Study the drawing (mm; zero at the part's minimum x, y, z) and answer. A direction names the side the tool comes from. Coordinates: 2 decimals unless noted, no trailing zeros. Order: outer loops, then holes, each group sorted by start corner. A loop starts at its lowest first (then second) coordinate and runs counter-clockwise, first axis right, second up. Notation, with made-up numbers: (54.25, 64) -> (69.25, 64) arc R16 cw to (69.25, 74) -> close; hole circle Ø10 at (34, -16). An arc over 180 degrees is marked (long way). Answer as CSV lines item,"result". Start each with the question number.
Item 1: Section A-A (z = 33) is taken. Write down the section's boundary in (x, y).
Item 2: Section B-B (y = 6) is taken. Write down the section's boundary in (x, z).
Item 3: Which of the six approach directions +Z, -Z, +X, -X, +Y, -Y give full straight-line access (tool end or side, diameter ignored) to the marked faces 1 and 2?
Item 4: Straight lines are drawn through the part: L1, parallel to X at y = 7.75, z = 28; L2, parallel to Z at x = 66.5, y = 6.75; L3, parallel to X at y = 6, z = 43.5. For each, find the intervals that lie inside material, in ascending order.
Item 5: Section C-C (x = 39) is taken. Write down the section's boundary in (y, z).
Item 6: Each of these flat-tipped pins is pushed along its axis until it touches: pin 1 Ø1.5 at (y, z) = (8, 35.5) entering from -X; pin 2 Ø3 at (y, z) = (10, 8.5) entering from -X. Where does it stop, or does it pass through?
Item 7: Section D-D (z = 44) is taken. Write down the section's boundary in (x, y), then the cut area to 3 significant figures.
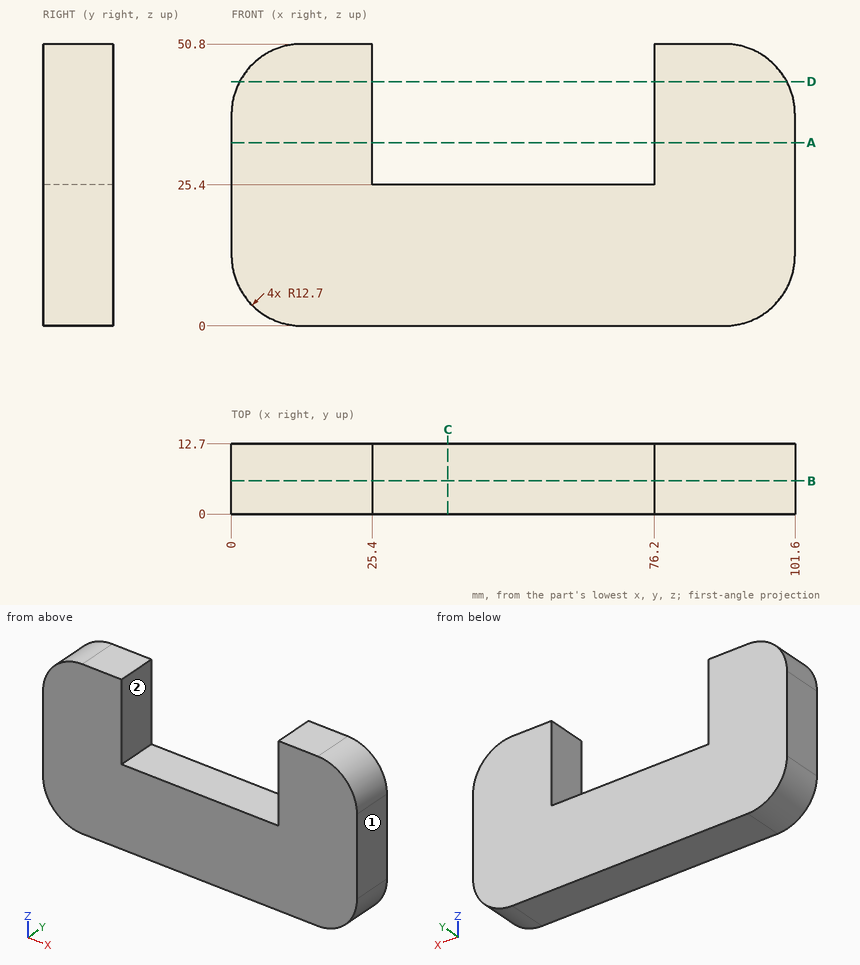
Checked values:
1,outline,"(0, 0) -> (25.4, 0) -> (25.4, 12.7) -> (0, 12.7) -> close; (76.2, 0) -> (101.6, 0) -> (101.6, 12.7) -> (76.2, 12.7) -> close"
2,outline,"(0, 12.7) arc R12.7 ccw to (12.7, 0) -> (88.9, 0) arc R12.7 ccw to (101.6, 12.7) -> (101.6, 38.1) arc R12.7 ccw to (88.9, 50.8) -> (76.2, 50.8) -> (76.2, 25.4) -> (25.4, 25.4) -> (25.4, 50.8) -> (12.7, 50.8) arc R12.7 ccw to (0, 38.1) -> close"
3,face 1,"+Z, -Z, +X, +Y, -Y"
3,face 2,"+Z, +Y, -Y"
4,L1,"x = 0 to 25.4, 76.2 to 101.6"
4,L2,"z = 0 to 25.4"
4,L3,"x = 1.21 to 25.4, 76.2 to 100.39"
5,outline,"(0, 0) -> (12.7, 0) -> (12.7, 25.4) -> (0, 25.4) -> close"
6,pin 1,"stops at x = 0"
6,pin 2,"stops at x = 0.29"
7,outline,"(1.45, 0) -> (25.4, 0) -> (25.4, 12.7) -> (1.45, 12.7) -> close; (76.2, 0) -> (100.15, 0) -> (100.15, 12.7) -> (76.2, 12.7) -> close"
7,area,"608 mm^2"
